Study the drawing (mm; zero at the part's minimum x, y, z) and answer. Coordinates: 2 decimals unless noted, no trailing zeros. Write each loop counter-clockwise with the first axis right and the second up, starting at its lowest first coordinate (ties: lowest second). Pieces come first, ordered by that corner, then holes. Notation, with made-up numbers: (0.25, 84) -> (15.25, 84) arc R16 cw to (15.25, 94) -> close; hole circle Ø1 at (36, 25). An arc over 180 degrees is marked (long way). Write item = value, one per line. Start each with the question number.
1) Section A-A (x = 10) is taken. Count the separate pieces of the cut face and the enclosed holes in it, plus the area to 3 significant figures.
2) For a pull along X with two mould halves and no side action, classify the marked faces 1, 2 and 3 as released by +X, released by -X, zero draft, split by the parting line, or undercut.
3) Section B-B (y = 23.5) is taken. Determine the outline of the cut face in (x, z), plus the area to 3 significant figures.
4) Flat-ended cylindrical pins translate along their axes: pin 1 Ø5 at (x, z) = (10, 10) entering from +Y; pin 2 Ø12 at (y, z) = (13, 6) entering from -X; pin 3 Ø1 at (x, y) = (7, 34.5) entering from -Z; pin 4 Ø8 at (y, z) = (20.5, 16.5) entering from +X. Find the tip coordinate at first contact, or state that the pin passes through.
5) Find the intervals of material crossed by line 1 along Y through (x, z) = (10, 14.5); line 2 along X through (y, z) = (26, 9.75); line 3 along Z through (x, y) = (10, 9), in increasing order. Write a range as from..to.
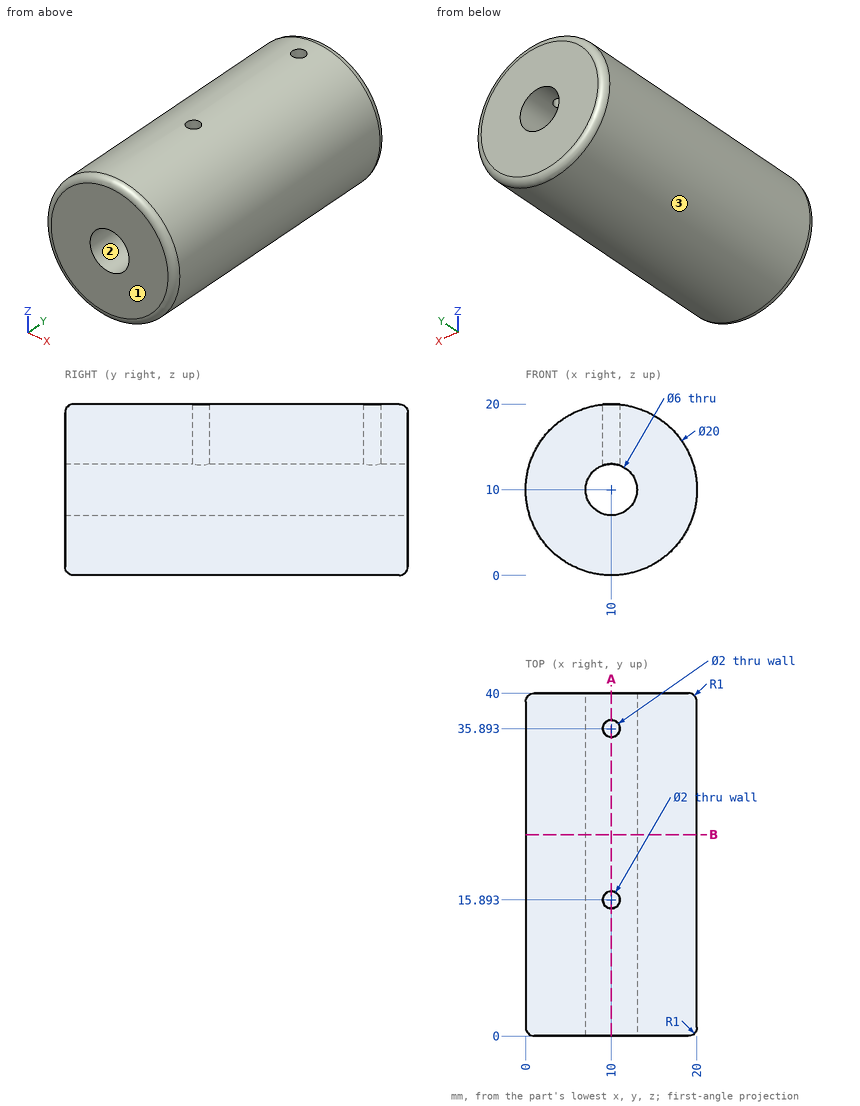
Answer key:
q1.separate_pieces = 4
q1.enclosed_holes = 0
q1.area = 531 mm^2
q2.face_1 = zero draft
q2.face_2 = undercut
q2.face_3 = split by the parting line
q3.outline = circle Ø20 at (10, 10); hole circle Ø6 at (10, 10)
q3.area = 286 mm^2
q4.pin_1 = through
q4.pin_2 = 0
q4.pin_3 = 0.32
q4.pin_4 = 19.68
q5.line_1 = 0..14.89, 16.89..34.89, 36.89..40
q5.line_2 = 0..7.01, 12.99..20
q5.line_3 = 0..7, 13..20
